Could you check a few things on this model? Use its own coordinates, in mm. A direction names the side the tool comes from. Round coordinates to 2 decimals unless told otherwise and drop trailing zeros. Write each question's results on one line, items separated by ' | '. Start each with the question number.
1) We'd pull the mould along Y, two halves only. Please class faces 3 (the cylindrical face through (-2.071, 32.048, 4.785)), 4 (the cylindrical face through (-48.89, 48.99, 3.13)), 5 (the flat face through (-1, -50.8, 3)): pulls with the +Y half, pulls with the -Y half, needs draft (parallel to the pull), parting line crosses it, or undercut.
2) If I drill on probe 1 along Y at (x, z) = (35, 3.75); probe 2 along Z at (x, y) = (32, -14.5) (3 decimals); probe 3 along Y at (x, z) = (-45.5, 0.75), over which ranges is the centre line in solid material (lowest first)?
3) Which directions (+Z, -Z, +X, -X, +Y, -Y) give clear straight access to the entire face, cutting with the end or side of a thin tool? Please do faces 1 (the cylindrical face through (-48.99, -48.89, 3.13)), 2 (the cylindrical face through (-31.83, 29.18, 4.78)).
from build123d import *

# Parameters (mm, degrees)
F1_DEPTH = 6.35
F2_R     = 43.18
F3_DEPTH = 3.175


with BuildPart() as f1:
    # F0 (on Top) → F1 (new body)
    with BuildSketch(Plane.XY):
        with BuildLine():
            Line((44.45, 50.8), (-44.45, 50.8))
            ThreePointArc((-44.45, 50.8), (-48.940128, 48.940128), (-50.8, 44.45))
            Line((-50.8, 44.45), (-50.8, -44.45))
            ThreePointArc((-50.8, -44.45), (-48.940128, -48.940128), (-44.45, -50.8))
            Line((-44.45, -50.8), (44.45, -50.8))
            ThreePointArc((44.45, -50.8), (48.940128, -48.940128), (50.8, -44.45))
            Line((50.8, -44.45), (50.8, 44.45))
            ThreePointArc((50.8, 44.45), (48.940128, 48.940128), (44.45, 50.8))
        make_face()
    extrude(amount=F1_DEPTH)

    # F2 (on face) → F3 (cut)
    with BuildSketch(Plane.XY.offset(6.35)):
        Circle(F2_R)
        with BuildLine():
            ThreePointArc((35.830027, -16.315821), (20.204607, -33.790098), (-2.58374, -39.285127))
            ThreePointArc((-2.58374, -39.285127), (4.747118, -36.517246), (10.782814, -31.519946))
            ThreePointArc((10.782814, -31.519946), (16.427451, -25.311935), (22.634907, -19.666689))
            ThreePointArc((22.634907, -19.666689), (29.030027, -17.194081), (35.830027, -16.315821))
        make_face(mode=Mode.SUBTRACT)
        with BuildLine():
            ThreePointArc((-9.899706, -38.105022), (-17.917908, -35.056319), (-25.085457, -30.343315))
            ThreePointArc((-25.085457, -30.343315), (-10.61459, -29.092618), (2.344406, -22.532538))
            ThreePointArc((2.344406, -22.532538), (9.787045, -15.731443), (17.303402, -9.011908))
            ThreePointArc((17.303402, -9.011908), (27.593343, -3.772844), (39.123036, -4.402834))
            ThreePointArc((39.123036, -4.402834), (38.232302, -9.396167), (36.706991, -14.233543))
            ThreePointArc((36.706991, -14.233543), (29.479665, -14.782685), (22.634907, -17.167022))
            ThreePointArc((22.634907, -17.167022), (15.458512, -22.677295), (9.168963, -29.181547))
            ThreePointArc((9.168963, -29.181547), (0.512727, -35.519703), (-9.899706, -38.105022))
        make_face(mode=Mode.SUBTRACT)
        with BuildLine():
            ThreePointArc((-28.951135, -26.680118), (-32.941202, -21.560939), (-36.035977, -15.855765))
            ThreePointArc((-36.035977, -15.855765), (-18.476277, -18.776194), (-2.58374, -10.757512))
            ThreePointArc((-2.58374, -10.757512), (4.205031, -5.018711), (10.782814, 0.960756))
            ThreePointArc((10.782814, 0.960756), (24.078577, 7.549898), (38.864055, 6.291432))
            ThreePointArc((38.864055, 6.291432), (39.291598, 2.483397), (39.34691, -1.348164))
            ThreePointArc((39.34691, -1.348164), (25.459159, -1.978206), (13.467762, -9.011908))
            ThreePointArc((13.467762, -9.011908), (5.843991, -16.249448), (-2.58374, -22.532538))
            ThreePointArc((-2.58374, -22.532538), (-15.275761, -27.732057), (-28.951135, -26.680118))
        make_face(mode=Mode.SUBTRACT)
        with BuildLine():
            ThreePointArc((-3.792618, -9.011908), (-20.108035, -16.966318), (-37.533355, -11.884619))
            ThreePointArc((-37.533355, -11.884619), (-39.334778, 1.664978), (-36.394785, 15.013879))
            ThreePointArc((-36.394785, 15.013879), (-19.548147, 17.120851), (-11.623084, 2.106128))
            ThreePointArc((-11.623084, 2.106128), (-15.8727, -6.927744), (-25.315939, -10.167394))
            ThreePointArc((-25.315939, -10.167394), (-32.018706, -6.233835), (-32.666095, 1.510897))
            ThreePointArc((-32.666095, 1.510897), (-27.765063, 6.938703), (-20.569334, 5.633835))
            ThreePointArc((-20.569334, 5.633835), (-18.810376, 0.630934), (-22.223454, -3.427865))
            ThreePointArc((-22.223454, -3.427865), (-24.636431, -3.441846), (-25.315939, -1.12648))
            ThreePointArc((-25.315939, -1.12648), (-24.87664, -0.443257), (-25.315939, 0.239966))
            ThreePointArc((-25.315939, 0.239966), (-26.550153, -0.620979), (-26.853859, -2.094843))
            ThreePointArc((-26.853859, -2.094843), (-24.8636, -4.486405), (-21.79506, -5.000961))
            ThreePointArc((-21.79506, -5.000961), (-18.057747, -1.44174), (-17.920237, 3.717394))
            ThreePointArc((-17.920237, 3.717394), (-25.512349, 9.134125), (-33.85007, 4.955185))
            ThreePointArc((-33.85007, 4.955185), (-35.104751, -1.829456), (-32.666095, -8.283798))
            ThreePointArc((-32.666095, -8.283798), (-24.810949, -12.292556), (-16.25191, -10.167394))
            ThreePointArc((-16.25191, -10.167394), (-11.765874, -4.942736), (-9.363333, 1.510897))
            ThreePointArc((-9.363333, 1.510897), (-1.52454, 0.163596), (5.813062, 3.233041))
            ThreePointArc((5.813062, 3.233041), (9.821154, 7.902724), (11.248579, 13.888808))
            ThreePointArc((11.248579, 13.888808), (15.748865, 11.857558), (20.686024, 11.802628))
            ThreePointArc((20.686024, 11.802628), (21.955711, 12.195598), (23.115785, 12.844257))
            ThreePointArc((23.115785, 12.844257), (28.022683, 20.770437), (25.723282, 29.804525))
            ThreePointArc((25.723282, 29.804525), (33.435684, 20.785858), (38.110449, 9.878793))
            ThreePointArc((38.110449, 9.878793), (23.134356, 10.130821), (9.823904, 3.26214))
            ThreePointArc((9.823904, 3.26214), (3.175845, -3.052608), (-3.792618, -9.011908))
        make_face(mode=Mode.SUBTRACT)
        with BuildLine():
            ThreePointArc((0, 20.890631), (-7.799723, 21.471197), (-13.435853, 16.048396))
            ThreePointArc((-13.435853, 16.048396), (-23.530574, 21.247029), (-34.610562, 18.764484))
            ThreePointArc((-34.610562, 18.764484), (-30.059834, 25.424462), (-24.247281, 31.017193))
            ThreePointArc((-24.247281, 31.017193), (-1.783652, 31.880624), (8.255853, 11.766737))
            ThreePointArc((8.255853, 11.766737), (1.823287, 3.295446), (-8.805102, 3.717394))
            ThreePointArc((-8.805102, 3.717394), (-9.814889, 8.75871), (-12.02473, 13.401031))
            ThreePointArc((-12.02473, 13.401031), (-5.439061, 19.784732), (2.594116, 15.358591))
            ThreePointArc((2.594116, 15.358591), (2.204285, 10.544215), (-2.272845, 8.73162))
            ThreePointArc((-2.272845, 8.73162), (-3.709614, 10.249179), (-2.272845, 11.766737))
            ThreePointArc((-2.272845, 11.766737), (-1.417286, 11.940645), (-1.321004, 12.808375))
            ThreePointArc((-1.321004, 12.808375), (-2.368046, 13.786265), (-3.799384, 13.724298))
            ThreePointArc((-3.799384, 13.724298), (-5.537072, 11.740216), (-5.199529, 9.124454))
            ThreePointArc((-5.199529, 9.124454), (-3.062346, 6.930124), (0, 6.861728))
            ThreePointArc((0, 6.861728), (4.041718, 10.566846), (4.168157, 16.048396))
            ThreePointArc((4.168157, 16.048396), (2.432702, 18.769606), (0, 20.890631))
        make_face(mode=Mode.SUBTRACT)
        with BuildLine():
            ThreePointArc((19.258106, 29.087057), (13.226177, 30.002315), (8.255853, 26.46427))
            ThreePointArc((8.255853, 26.46427), (-2.006518, 34.7072), (-15.063429, 36.374304))
            ThreePointArc((-15.063429, 36.374304), (4.607369, 39.099476), (23.105911, 31.87654))
            ThreePointArc((23.105911, 31.87654), (26.454351, 24.174835), (24.335554, 16.048396))
            ThreePointArc((24.335554, 16.048396), (17.630398, 13.197088), (10.830184, 15.813604))
            ThreePointArc((10.830184, 15.813604), (10.39549, 20.23006), (8.760267, 24.355602))
            ThreePointArc((8.760267, 24.355602), (11.335212, 27.319516), (15.109342, 28.40168))
            ThreePointArc((15.109342, 28.40168), (15.317869, 28.40325), (15.526231, 28.411666))
            ThreePointArc((15.526231, 28.411666), (19.698978, 26.851735), (21.36774, 22.721307))
            ThreePointArc((21.36774, 22.721307), (19.997953, 20.134608), (17.147247, 19.470681))
            ThreePointArc((17.147247, 19.470681), (16.193526, 20.763747), (17.147247, 22.056814))
            ThreePointArc((17.147247, 22.056814), (17.406668, 23.306557), (16.141526, 23.475597))
            ThreePointArc((16.141526, 23.475597), (14.803341, 21.221821), (15.323924, 18.652923))
            ThreePointArc((15.323924, 18.652923), (18.345832, 17.155036), (21.36774, 18.652923))
            ThreePointArc((21.36774, 18.652923), (22.886635, 24.390358), (19.258106, 29.087057))
        make_face(mode=Mode.SUBTRACT)
    extrude(amount=-F3_DEPTH, mode=Mode.SUBTRACT)


solid = f1.part
Checked values:
1) face 3: undercut | face 4: pulls with the +Y half | face 5: pulls with the -Y half
2) probe 1: -50.8 to -25.29, -18.03 to -16.33, -14.19 to -3.47, -0.82 to 7.42, 10.55 to 18.03, 25.29 to 50.8 | probe 2: 0 to 3.175 | probe 3: -50.71 to 50.71
3) face 1: +Z, -Z, -X, -Y | face 2: +Z
